Geometry check sheet. Reference: drawing and pictorial views, mm from the part's lowest x, y, z. Round coordinates to 2 decimals unless told otherwise and drop trailing zeros. Write each loop counter-clockwise with the first axis right and the second up, starting at its lowest first coordinate (ties: lowest second). Pieces come first, ordered by that corner, then holes. Notation, with made-up numbers: (37, 25) -> (72, 25) arc R28 ccw to (72, 61) -> close; hole circle Ø4 at (34, 55). An arc over 180 degrees is marked (long way). Answer as a JSON object with one key per item and string values. Group by question number.
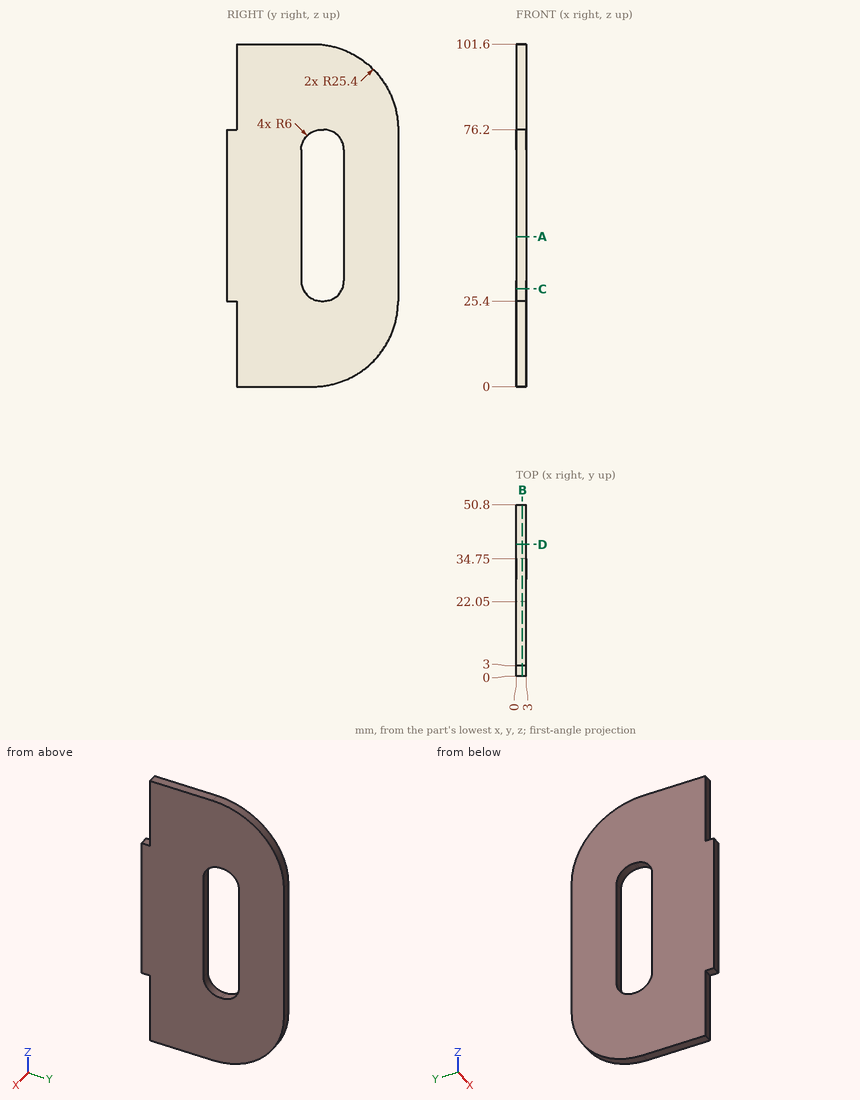
(1) Go/stop test with flat-tipped pins: pin 1 Ø0.9 at (x, y) = (2, 1) entering from -Z; pin 2 Ø1.5 at (x, y) = (1, 34.5) entering from -Z. Record where each tip stops, or that it passes through.
(2) Section check D-D on y = 39. Record the cut outline in (x, z).
(3) Section check B-B on x = 1.85. Record the cut outline in (y, z).
(4) Section check A-A on z = 44.5. Record the cut outline in (x, y).
(5) Section check C-C on z = 29. Record the cut outline in (x, y), then the cut area to 3 significant figures.
(6) Scan lines: line 1 along Y through (x, z) = (1.8, 63); line 2 along Z through (x, y) = (1.6, 31.5); line 3 along Z through (x, y) = (2.3, 46). Record each from-to range of solid material in increasing order.
Data:
{
 "1": {"pin 1": "stops at z = 25.4", "pin 2": "stops at z = 1.41"},
 "2": {"outline": "(0, 3.95) -> (3, 3.95) -> (3, 97.65) -> (0, 97.65) -> close"},
 "3": {"outline": "(0, 25.4) -> (3, 25.4) -> (3, 0) -> (25.4, 0) arc R25.4 ccw to (50.8, 25.4) -> (50.8, 76.2) arc R25.4 ccw to (25.4, 101.6) -> (3, 101.6) -> (3, 76.2) -> (0, 76.2) -> close; hole (22.05, 31.4) arc R6 ccw to (28.05, 25.4) -> (28.75, 25.4) arc R6 ccw to (34.75, 31.4) -> (34.75, 70.2) arc R6 ccw to (28.75, 76.2) -> (28.05, 76.2) arc R6 ccw to (22.05, 70.2) -> close"},
 "4": {"outline": "(0, 0) -> (3, 0) -> (3, 22.05) -> (0, 22.05) -> close; (0, 34.75) -> (3, 34.75) -> (3, 50.8) -> (0, 50.8) -> close"},
 "5": {"outline": "(0, 0) -> (3, 0) -> (3, 22.55) -> (0, 22.55) -> close; (0, 34.25) -> (3, 34.25) -> (3, 50.8) -> (0, 50.8) -> close", "area": "117 mm²"},
 "6": {"line 1": "y = 0 to 22.05, 34.75 to 50.8", "line 2": "z = 0.74 to 26.07, 75.53 to 100.86", "line 3": "z = 10.54 to 91.06"}
}
